The model under review builds one solid part; all positions refer to its coordinate system, in mm. Round coordinates to 2 decimals unless told otherwise and drop trailing zeros. Order: outer loops, then holes, each group sorted by start corner. A loop starts at its lowest first (then second) coordinate and runs counter-clockwise, first axis right, second up.
1) Consider section B-B (y = -59.5). Give the boundary of the cut face in (x, z) (3 decimals).
2) To check wall thickness, follow L1, parallel to X at y = 0, z = 45 (3 decimals); L2, parallel to Y at x = 4.25, z = 46.5; L3, parallel to Y at x = 0, z = 28 (3 decimals). State the ranges of each line that lie inside material, in increasing order.
3) Clearance check with flat-ended pins moving along their axes: P1, Ø4, axis at y = -62, z = 10, coming from the -X side (3 decimals); P2, Ø4, axis at x = 0, y = 0, coming from the +Z side; P3, Ø1.5, axis at x = 1, z = 38.5, coming from the -Y side; P4, Ø6, axis at x = -3.5, z = 55, coming from the -Y side. State where each tip first meets the part, or that it passes through.
4) Consider section A-A (z = 48.5). Give the boundary of the cut face in (x, y) (3 decimals), then the cut area to 3 significant figures.
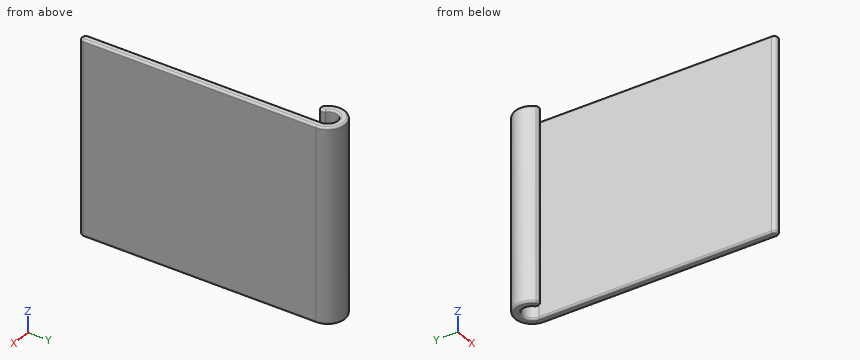
from build123d import *

# Parameters (mm, degrees)
BOSS_EXTRUDE1_DEPTH = 63.5
FILLET1_R           = 0.635


with BuildPart() as part:
    # Sketch1 → Boss-Extrude1 (new body)
    with BuildSketch(Plane.XY):
        with BuildLine():
            Line((3.175, 0), (3.175, -76.2))
            ThreePointArc((3.175, -76.2), (4.445, -77.47), (5.715, -76.2))
            Line((5.715, -76.2), (5.715, 0))
            ThreePointArc((5.715, 0), (-2.187035816, 5.279971528), (-4.041115254, -4.041115254))
            ThreePointArc((-4.041115254, -4.041115254), (-2.24506403, -4.041115254), (-2.24506403, -2.24506403))
            ThreePointArc((-2.24506403, -2.24506403), (-1.215019898, 2.933317516), (3.175, 0))
        make_face()
    extrude(amount=BOSS_EXTRUDE1_DEPTH)

    # Fillet1
    fillet1_edges = [part.edges().sort_by_distance(p)[0] for p in [
        (-2.187035816, 5.279971528, 63.5),
        (-2.24506403, -4.041115254, 63.5),
        (-1.215019898, 2.933317516, 63.5),
        (3.175, -38.1, 63.5),
        (4.445, -77.47, 63.5),
        (3.175, -38.1, 0),
        (-1.215019898, 2.933317516, 0),
        (-2.24506403, -4.041115254, 0),
        (5.715, -38.1, 63.5),
        (-2.187035816, 5.279971528, 0),
        (5.715, -38.1, 0),
        (4.445, -77.47, 0),
    ]]
    fillet(fillet1_edges, radius=FILLET1_R)


solid = part.part
Answer below:
1. outline: (3.175, 0.635) arc R0.635 ccw to (3.81, 0) - (5.08, 0) arc R0.635 ccw to (5.715, 0.635) - (5.715, 62.865) arc R0.635 ccw to (5.08, 63.5) - (3.81, 63.5) arc R0.635 ccw to (3.175, 62.865) - close
2. L1: x = -5.715 to -3.175, 3.175 to 5.715
2. L2: y = -77.45 to 3.82
2. L3: y = 3.175 to 5.715
3. P1: stops at x = 3.175
3. P2: passes through
3. P3: stops at y = 2.65
3. P4: stops at y = -4.41
4. outline: (-4.041, -4.041) arc R1.27 ccw to (-2.245, -2.245) arc R3.175 cw (long way) to (3.175, 0) - (3.175, -76.2) arc R1.27 ccw to (5.715, -76.2) - (5.715, 0) arc R5.715 ccw (long way) to start
4. area: 243 mm2
